Autodesk Inventor part; units mm, degrees
ref_plane "Work Plane1" through (-29.8485, -37.5485, 6) normal (0, 0, 1) x (1, 0, 0)
ref_plane "Work Plane3" through (-29.8485, -37.5485, 8) normal (0, 0, 1) x (1, 0, 0)
ref_plane "Work Plane2" through (-27.235, -34.935, 21) normal (0, 0, 1) x (1, 0, 0)
sketch "Sketch1" plane through (0, 0, 0) normal (0, 0, 1) x (1, 0, 0)
  circle A0 centre (0, -7.7) radius 6 construction
  circle A1 centre (18.5, -7.7) radius 2.4 construction
  circle A2 centre (-18.5, -7.7) radius 2.4 construction
  circle A3 centre (0, 12.9) radius 2 construction
  circle A4 centre (-31.7, -20.7) radius 2 construction
  circle A5 centre (31.7, -20.7) radius 2 construction
  circle A6 centre (31.7, 20.7) radius 2 construction
  circle A7 centre (-31.7, 20.7) radius 2 construction
  line L0 (-36.7, -25.7) -> (36.7, -25.7) construction
  line L1 (36.7, -25.7) -> (36.7, 25.7) construction
  line L2 (36.7, 25.7) -> (-36.7, 25.7) construction
  line L3 (-36.7, 25.7) -> (-36.7, -25.7) construction
  circle A8 centre (-31.7, 20.7) radius 3
  circle A9 centre (31.7, 20.7) radius 3
  circle A10 centre (31.7, -20.7) radius 3
  circle A11 centre (-31.7, -20.7) radius 3
  circle A12 centre (-31.7, 20.7) radius 5
  circle A13 centre (31.7, 20.7) radius 5
  circle A14 centre (31.7, -20.7) radius 5
  circle A15 centre (-31.7, -20.7) radius 5
  circle A16 centre (0, -7.7) radius 11
  line L4 (-30.6423, -25.5868) -> (2.3269, -18.4511)
  line L5 (-2.3269, -18.4511) -> (30.6423, -25.5868)
  line L6 (34.378, -16.4776) -> (5.8915, 1.5893)
  line L7 (-34.378, -16.4776) -> (-5.8915, 1.5893)
  line L8 (-28.9219, 24.8572) -> (6.1117, 1.4459)
  line L9 (-35.5281, 17.4835) -> (-8.4217, -14.7764)
  line L10 (-6.1117, 1.4459) -> (28.9219, 24.8572)
  line L11 (35.5281, 17.4835) -> (8.4217, -14.7764)
  circle A17 centre (0, -7.7) radius 9
  point P0 (0, 0)
  dimension "d0" = 1
  dimension "d1" = 2
  dimension "d2" = 5
  dimension "d3" = 3
extrude "Extrusion1" add sketch "Sketch1" along normal blind 4
ref_plane "Work Plane1" through (-29.8485, -37.5485, 6) normal (0, 0, 1) x (1, 0, 0)
ref_plane "Work Plane3" through (-29.8485, -37.5485, 8) normal (0, 0, 1) x (1, 0, 0)
sketch "Sketch2" plane through (0, 0, 4) normal (0, 0, 1) x (1, 0, 0)
  circle A0 centre (0, -7.7) radius 28.486 construction
  circle A1 centre (31.7, -20.7) radius 3 construction
  line L0 (0, -18.9547) -> (30.6423, -25.5868) construction
  arc A2 (30.6423, -25.5868) -> (34.378, -16.4776) centre (31.7, -20.7) ccw construction
  line L1 (34.378, -16.4776) -> (16.5128, -5.147) construction
  line L2 (16.5128, -5.147) -> (35.5281, 17.4835) construction
  arc A3 (35.5281, 17.4835) -> (28.9219, 24.8572) centre (31.7, 20.7) ccw construction
  line L3 (28.9219, 24.8572) -> (0, 5.53) construction
  line L4 (0, 5.53) -> (-28.9219, 24.8572) construction
  arc A4 (-28.9219, 24.8572) -> (-35.5281, 17.4835) centre (-31.7, 20.7) ccw construction
  line L5 (-35.5281, 17.4835) -> (-16.5128, -5.147) construction
  line L6 (-16.5128, -5.147) -> (-34.378, -16.4776) construction
  arc A5 (-34.378, -16.4776) -> (-30.6423, -25.5868) centre (-31.7, -20.7) ccw construction
  line L7 (-30.6423, -25.5868) -> (0, -18.9547) construction
  circle A6 centre (0, -7.7) radius 9 construction
  circle A7 centre (-31.7, -20.7) radius 3 construction
  circle A8 centre (-31.7, 20.7) radius 3 construction
  circle A9 centre (31.7, 20.7) radius 3 construction
  line L8 (0, -7.7) -> (31.7, 20.7) construction
  line L9 (0, -7.7) -> (-31.7, 20.7) construction
  circle A10 centre (23.2277, 13.1097) radius 2.7 construction
  circle A11 centre (-23.2277, 13.1097) radius 2.7 construction
  circle A12 centre (-23.2277, 13.1097) radius 2.5
  circle A13 centre (23.2277, 13.1097) radius 2.5
  point P0 (0, 0)
  dimension "d7" = 0.2
  dimension "d8" = 5
extrude "Extrusion2" add sketch "Sketch2" along normal up to surface (4 mm away)
sketch "Sketch5" plane through (0, 0, 4) normal (0, 0, 1) x (1, 0, 0)
  circle A0 centre (-23.2277, 13.1097) radius 2.5 construction
  circle A1 centre (23.2277, 13.1097) radius 2.5 construction
  circle A2 centre (31.7, -20.7) radius 3 construction
  line L0 (0, -18.9547) -> (30.6423, -25.5868)
  arc A3 (30.6423, -25.5868) -> (34.378, -16.4776) centre (31.7, -20.7) ccw
  line L1 (34.378, -16.4776) -> (16.5128, -5.147) construction
  line L2 (16.5128, -5.147) -> (35.5281, 17.4835) construction
  arc A4 (35.5281, 17.4835) -> (28.9219, 24.8572) centre (31.7, 20.7) ccw
  line L3 (28.9219, 24.8572) -> (0, 5.53)
  line L4 (0, 5.53) -> (-28.9219, 24.8572)
  arc A5 (-28.9219, 24.8572) -> (-35.5281, 17.4835) centre (-31.7, 20.7) ccw
  line L5 (-35.5281, 17.4835) -> (-16.5128, -5.147) construction
  line L6 (-16.5128, -5.147) -> (-34.378, -16.4776) construction
  arc A6 (-34.378, -16.4776) -> (-30.6423, -25.5868) centre (-31.7, -20.7) ccw
  line L7 (-30.6423, -25.5868) -> (0, -18.9547)
  circle A7 centre (0, -7.7) radius 9 construction
  circle A8 centre (-31.7, -20.7) radius 3 construction
  circle A9 centre (-31.7, 20.7) radius 3 construction
  circle A10 centre (31.7, 20.7) radius 3 construction
  line L8 (16.5128, -5.147) -> (-16.5128, -5.147) construction
  line L9 (0, -18.9547) -> (0, 5.53) construction
  line L10 (-25, 25.853) -> (-25, -36.147)
  line L11 (-25, -36.147) -> (25, -36.147)
  line L12 (25, -36.147) -> (25, 25.853)
  line L13 (25, 25.853) -> (-25, 25.853)
  line L14 (-25, 25.853) -> (25, -36.147) construction
  line L15 (-25, -36.147) -> (25, 25.853) construction
  circle A11 centre (0, -7.7) radius 9
  circle A12 centre (0, -7.7) radius 9
  line L16 (-25, -36.147) -> (-35.4893, -23.962)
  arc A13 (-34.378, -16.4776) -> (-30.6423, -25.5868) centre (-31.7, -20.7) ccw
  line L17 (25, -36.147) -> (35.4893, -23.962)
  arc A14 (30.6423, -25.5868) -> (34.378, -16.4776) centre (31.7, -20.7) ccw
  line L18 (-25, 25.853) -> (-31.8132, 25.6987)
  arc A15 (-28.9219, 24.8572) -> (-35.5281, 17.4835) centre (-31.7, 20.7) ccw
  line L19 (25, 25.853) -> (31.8132, 25.6987)
  arc A16 (35.5281, 17.4835) -> (28.9219, 24.8572) centre (31.7, 20.7) ccw
  point P0 (0, 0)
  point P1 (0, -5.147)
  dimension "d17" = 62
  dimension "d18" = 50
extrude "Extrusion5" add sketch "Sketch5" against normal up to surface (4 mm away)
sketch "Sketch4" plane through (0, 0, 4) normal (0, 0, 1) x (1, 0, 0)
  circle A0 centre (-18.5, -7.7) radius 2.4 construction
  circle A1 centre (18.5, -7.7) radius 2.4 construction
  circle A2 centre (18.5, -7.7) radius 2.9
  circle A3 centre (-18.5, -7.7) radius 2.9
  point P0 (0, 0)
  dimension "d14" = 0.5
extrude "Extrusion4" cut sketch "Sketch4" against normal up to surface (4 mm away)
sketch "Sketch6" plane through (0, 0, 4) normal (0, 0, 1) x (1, 0, 0)
  circle A0 centre (18.5, -7.7) radius 2.9 construction
  circle A1 centre (-18.5, -7.7) radius 2.9 construction
  circle A2 centre (-31.7, -20.7) radius 3 construction
  circle A3 centre (-31.7, 20.7) radius 3 construction
  circle A4 centre (0, -7.7) radius 9 construction
  circle A5 centre (31.7, 20.7) radius 3 construction
  arc A6 (35.4893, -23.962) -> (34.378, -16.4776) centre (31.7, -20.7) ccw construction
  line L0 (34.378, -16.4776) -> (25, -10.5299) construction
  line L1 (25, -10.5299) -> (25, 4.9538) construction
  line L2 (25, 4.9538) -> (35.5281, 17.4835) construction
  arc A7 (35.5281, 17.4835) -> (31.8132, 25.6987) centre (31.7, 20.7) ccw construction
  line L3 (25, 25.853) -> (-25, 25.853) construction
  arc A8 (-31.8132, 25.6987) -> (-35.5281, 17.4835) centre (-31.7, 20.7) ccw construction
  line L4 (-35.5281, 17.4835) -> (-25, 4.9538) construction
  line L5 (-25, 4.9538) -> (-25, -10.5299) construction
  line L6 (-25, -10.5299) -> (-34.378, -16.4776) construction
  arc A9 (-34.378, -16.4776) -> (-35.4893, -23.962) centre (-31.7, -20.7) ccw construction
  line L7 (-25, -36.147) -> (25, -36.147) construction
  circle A10 centre (31.7, -20.7) radius 3 construction
  line L8 (0, -7.7) -> (31.7, -20.7) construction
  line L9 (0, -7.7) -> (-31.7, -20.7) construction
  circle A11 centre (23.2277, 13.1097) radius 2.5
  line L10 (31.8132, 25.6987) -> (25, 25.853)
  line L11 (-25, 25.853) -> (-31.8132, 25.6987)
  line L12 (-35.4893, -23.962) -> (-25, -36.147)
  line L13 (25, -36.147) -> (35.4893, -23.962)
  circle A12 centre (23.2277, 13.1097) radius 2.5
  circle A13 centre (-23.2277, 13.1097) radius 2.5
  circle A14 centre (17.4777, -33.5282) radius 2.5
  circle A15 centre (0, -7.7) radius 31.186 construction
  circle A16 centre (-17.4777, -33.5282) radius 2.5
  circle A17 centre (-23.2277, 13.1097) radius 2.5
  arc A18 (19.1487, 13.5246) -> (-19.1487, 13.5246) centre (0, -7.7) ccw
  arc A19 (-19.2697, 12.04) -> (-19.1487, 13.5246) centre (-23.2277, 13.1097) ccw
  arc A20 (19.2697, 12.04) -> (-19.2697, 12.04) centre (0, -7.7) ccw
  arc A21 (19.1487, 13.5246) -> (19.2697, 12.04) centre (23.2277, 13.1097) ccw
  point P0 (0, 0)
  point P1 (23.7277, 10.2129)
  point P2 (20.4031, 13.9239)
  dimension "d25" = 5.75
  dimension "d26" = 0
ref_plane "Work Plane2" through (-27.235, -34.935, 21) normal (0, 0, 1) x (1, 0, 0)
extrude "Extrusion6" add sketch "Sketch6" along normal up to surface (4 mm away) contours A14 | A16
chamfer "Chamfer1" distance 0.5 angle 45 4 edges at (-25.7277, 13.1097, 4) (20.7277, 13.1097, 4) (14.9777, -33.5282, 4) (-19.9777, -33.5282, 4)
properties part number "adpaterPlate"
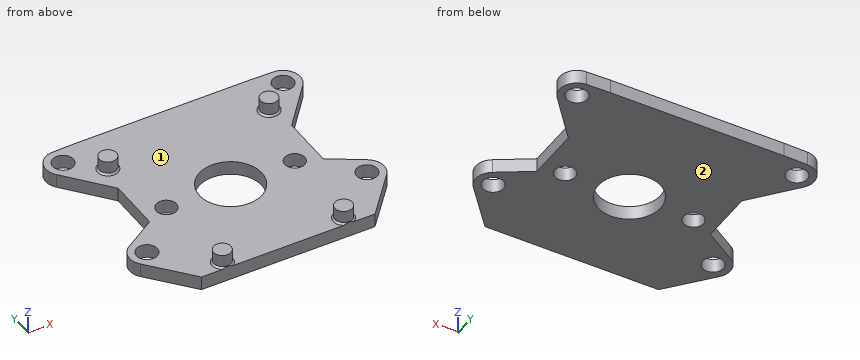
Can you work these out from the model? Positions are in its coordinate system, mm. Face numbers are marked on the shaded views. Coordinates: 2 decimals unless noted, no trailing zeros. Loops run counter-clockwise (first coordinate to the right, second up) from the corner with the lowest first, then second, coordinate; pieces in that order, holes last. Notation, with made-up numbers: (70, 25.5) - (83, 25.5) arc R27 cw to (83, 53.5) - close; hole circle Ø4 at (83, 17.25). An arc over 180 degrees is marked (long way). Use a Markdown table: item, result.
Item 1: I want a section at C-C on z = 2. Please give me the cut outline in (x, y).
Numbers:
| item | result |
|---|---|
| outline | (-35.53, 17.48) - (-25, 4.95) - (-25, -10.53) - (-34.38, -16.48) arc R5 ccw to (-35.49, -23.96) - (-25, -36.15) - (25, -36.15) - (35.49, -23.96) arc R5 ccw to (34.38, -16.48) - (25, -10.53) - (25, 4.95) - (35.53, 17.48) arc R5 ccw to (31.81, 25.7) - (25, 25.85) - (-25, 25.85) - (-31.81, 25.7) arc R5 ccw to start; hole circle Ø6 at (-31.7, -20.7); hole circle Ø6 at (-31.7, 20.7); hole circle Ø5.8 at (-18.5, -7.7); hole circle Ø18 at (0, -7.7); hole circle Ø5.8 at (18.5, -7.7); hole circle Ø6 at (31.7, -20.7); hole circle Ø6 at (31.7, 20.7) |
Item 2: I want a section at D-D on x = -11. Please give me the cut outline in (y, z), and give its area (3 significant figures).
Numbers:
| item | result |
|---|---|
| outline | (-36.15, 0) - (25.85, 0) - (25.85, 4) - (-36.15, 4) - close |
| area | 248 mm2 |
Item 3: We'd pull the mould along X, two halves only. Please class the marked faces 1 and 2: released by +X, released by -X, zero draft, split by the parting line, or undercut.
Numbers:
| item | result |
|---|---|
| face 1 | undercut |
| face 2 | zero draft |
Item 4: Will these pins go through, and if not, where does the flat tip stop? pin 1 (2 mm diameter, centred on x = 22, y = -24.5, fed in from -Z); pin 2 (3 mm diameter, centred on x = -29, z = 3.5, fed in from +Y); pin 3 (7 mm diameter, centred on x = -31.7, y = -20.7, fed in from +Z); pin 4 (3 mm diameter, centred on y = -1, z = 3, fed in from -X).
Numbers:
| item | result |
|---|---|
| pin 1 | stops at z = 0 |
| pin 2 | stops at y = 25.8 |
| pin 3 | stops at z = 4 |
| pin 4 | stops at x = -25 |
Item 5: I want a section at B-B on x = 0. Please give me the cut outline in (y, z), and give its area (3 significant figures).
Numbers:
| item | result |
|---|---|
| outline | (-36.15, 0) - (-16.7, 0) - (-16.7, 4) - (-36.15, 4) - close; (1.3, 0) - (25.85, 0) - (25.85, 4) - (1.3, 4) - close |
| area | 176 mm2 |
Item 6: I want a section at A-A on y = -7.7. Please give me the cut outline in (x, z), and give its area (3 significant figures).
Numbers:
| item | result |
|---|---|
| outline | (-25, 0) - (-21.4, 0) - (-21.4, 4) - (-25, 4) - close; (-15.6, 0) - (-9, 0) - (-9, 4) - (-15.6, 4) - close; (9, 0) - (15.6, 0) - (15.6, 4) - (9, 4) - close; (21.4, 0) - (25, 0) - (25, 4) - (21.4, 4) - close |
| area | 81.6 mm2 |
Item 7: If I drill on probe 1 along Y at (x, z) = (18.5, 2.8); probe 2 along Y at (x, z) = (0, 1.9); probe 3 along Y at (x, z) = (-29, 2), over which ranges is the centre line in solid material (lowest first)? Write a range as from..to.
Numbers:
| item | result |
|---|---|
| probe 1 | y = -36.15..-10.6, -4.8..25.85 |
| probe 2 | y = -36.15..-16.7, 1.3..25.85 |
| probe 3 | y = -31.5..-22.01, -19.39..-13.07, 9.71..19.39, 22.01..25.76 |
